The drawing under review shows one solid part. Ordinate dimensions are in mm from its lowest x, y, z. A direction names the side the tool comes from. Give positions to 0.01 mm unless a question says otherwise; leave off trailing zeros. Order: outer loops, then holes, each group sorted by start corner. A loop starts at its lowest first (then second) coordinate and runs counter-clockwise, first axis right, second up. Notation, with made-up numbers: (8.25, -40) - (61.25, -40) arc R30 cw to (61.25, -12) - close; hole circle Ø10 at (-7, -21.75). An arc over 180 degrees is marked (long way). Use CSV: the item, a comma, the result in double quotes. Start each with the question number.
1. Take a section at D-D, the plane y = 82.5. State the section outline as (x, z) points, then the cut area to 3 significant figures.
2. To check wall thickness, follow line 1 (Y direction, x = 136, z = 20); line 2 (Y direction, x = 181.5, z = 10.5); line 3 (X direction, y = 65, z = 11). State the ranges of each line that lie inside material, in increasing order. Write a range as [from, to].
3. For pin 1 (4 mm diameter, centred on x = 197.5, y = 45, fed in from -Z); pin 2 (24 mm diameter, centred on y = 57.5, z = 20, fed in from -X); pin 3 (9.5 mm diameter, centred on y = 53, z = 20, fed in from +X); pin 4 (12 mm diameter, centred on x = 148, z = 20, fed in from -Y), all flat-tipped, find the tip position at first contact; note any pin that passes through.
4. Take a section at B-B, the plane y = 53. State the section outline as (x, z) points.
5. Take a section at C-C, the plane x = 175. State the section outline as (y, z) points.
6. Machinability: for the marked faces 1, 2 and 3, which of the approach directions +Z, -Z, +X, -X, +Y, -Y give a long, thin tool a straight path to every point of the face, cutting with its end or side? Answer none if there is none.
7. Take a section at A-A, the plane z = 20. State the section outline as (x, y) points, then the cut area to 3 significant figures.
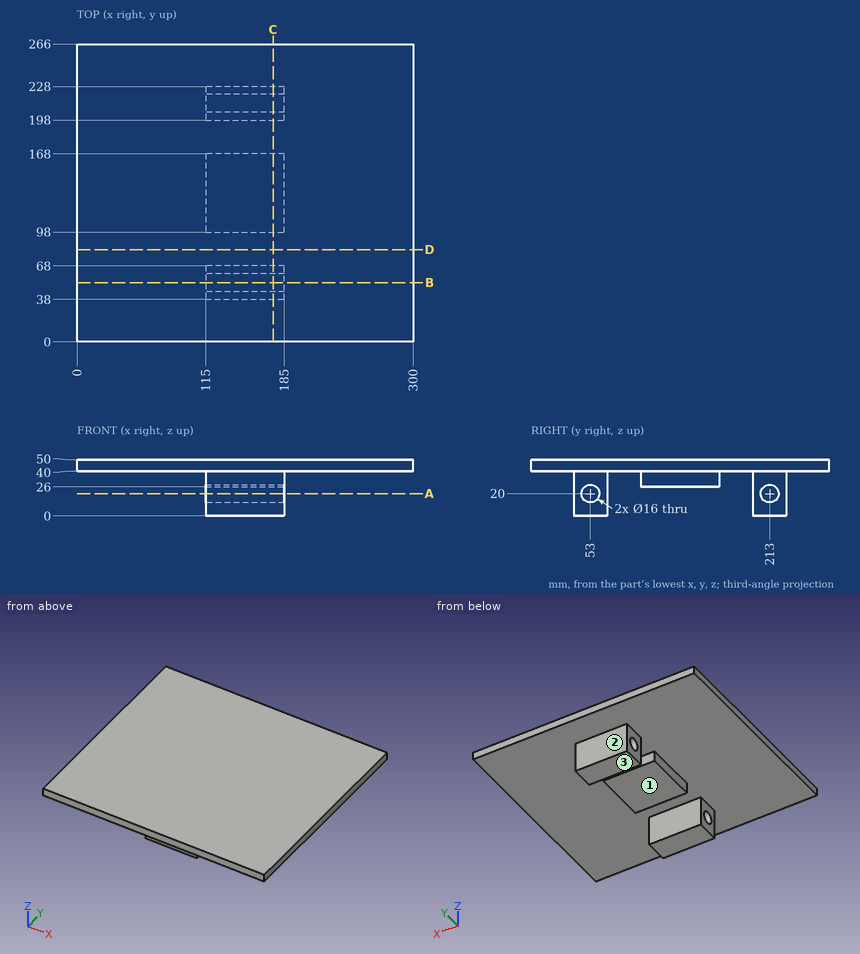
Determined:
1,outline,"(0, 40) - (300, 40) - (300, 50) - (0, 50) - close"
1,area,"3,000 mm²"
2,line 1,"y = [38, 45], [61, 68], [198, 205], [221, 228]"
2,line 2,"y = [38, 68], [198, 228]"
2,line 3,"x = [115, 185]"
3,pin 1,"stops at z = 40"
3,pin 2,"stops at x = 115"
3,pin 3,"passes through"
3,pin 4,"stops at y = 38"
4,outline,"(0, 40) - (115, 40) - (115, 28) - (185, 28) - (185, 40) - (300, 40) - (300, 50) - (0, 50) - close; (115, 0) - (185, 0) - (185, 12) - (115, 12) - close"
5,outline,"(0, 40) - (38, 40) - (38, 0) - (68, 0) - (68, 40) - (98, 40) - (98, 26) - (168, 26) - (168, 40) - (198, 40) - (198, 0) - (228, 0) - (228, 40) - (266, 40) - (266, 50) - (0, 50) - close; hole circle Ø16 at (53, 20); hole circle Ø16 at (213, 20)"
6,face 1,"-Z, +X, -X"
6,face 2,"-Z, +X, -X, +Y"
6,face 3,"-Z, +X, -X, +Y, -Y"
7,outline,"(115, 38) - (185, 38) - (185, 45) - (115, 45) - close; (115, 61) - (185, 61) - (185, 68) - (115, 68) - close; (115, 198) - (185, 198) - (185, 205) - (115, 205) - close; (115, 221) - (185, 221) - (185, 228) - (115, 228) - close"
7,area,"1,960 mm²"
